```python
from build123d import *

# Parameters (mm, degrees)
EXTRUDE_5_DEPTH = 5.5


with BuildPart() as part:
    # Эскиз1 → Бобышка-Вытянуть5 (new body)
    with BuildSketch(Plane(origin=(0, 0, 0), x_dir=(0, 0, -1), z_dir=(1, 0, 0))):
        Polygon((0.00204272, 35), (0.00204272, 0.000377999), (35.00204272, 0.000377999), (35.00204272, 5.000377999), (70, 5.000377999), (70, 0.000377999), (105.00204272, 0.000377999), (105.00204272, 5.000377999), (140, 5.000377999), (140, 0.000377999), (170, 0.000377999), (170, 35.000377999), (175, 35.000377999), (175, 70), (170, 70), (170, 105.000377999), (175, 105.000377999), (175, 140), (170, 140), (170, 170.000377999), (140.00204272, 170.000377999), (140.00204272, 175.000377999), (139.90204272, 175.000377999), (105, 175.000377999), (105, 170.000377999), (70.00204272, 170.000377999), (70.00204272, 175.000377999), (35, 175.000377999), (35, 170.000377999), (0.00204272, 170.000377999), (0.00204272, 140.000377999), (5.00204272, 140.000377999), (5.00204272, 105), (0.00204272, 105), (0.00204272, 70.000377999), (5.00204272, 70.000377999), (5.00204272, 35), align=None)
        Polygon((71.614687911, 65.697512044), (117.541103017, 19.771096938), (25.688272806, 19.771096938), align=None, mode=Mode.SUBTRACT)
        Polygon((20.031418556, 82.648268821), (48.641577373, 54.038110004), (20.031418556, 25.427951188), align=None, mode=Mode.SUBTRACT)
        Polygon((100.61937762, 42.349676584), (131.978534805, 73.708833769), (155.00204272, 50.685325854), (155.00204272, 19.771096938), (123.197957266, 19.771096938), align=None, mode=Mode.SUBTRACT)
        Polygon((105.802272221, 99.885096353), (129.15010768, 76.537260894), (97.790950495, 45.178103709), (74.443115036, 68.525939168), align=None, mode=Mode.SUBTRACT)
        Polygon((20.031418556, 150.499080414), (82.56698317, 87.963515801), (51.470004498, 56.866537129), (20.031418556, 88.30512307), align=None, mode=Mode.SUBTRACT)
        Polygon((84.688303513, 154.741721101), (117.016745992, 122.413278623), (86.809623857, 92.206156488), (24.274059243, 154.741721101), align=None, mode=Mode.SUBTRACT)
        Polygon((108.630699345, 102.713523478), (155.00204272, 149.084866852), (155.00204272, 56.342180104), align=None, mode=Mode.SUBTRACT)
        Polygon((149.34518847, 154.741721101), (119.845173116, 125.241705748), (90.345157763, 154.741721101), align=None, mode=Mode.SUBTRACT)
    extrude(amount=EXTRUDE_5_DEPTH)


solid = part.part
```
Geometry check sheet. Reference: the model listing, model coordinates, mm. A direction names the side the tool comes from. Coordinates: 2 decimals unless noted, no trailing zeros. Loops run counter-clockwise (first coordinate to the right, second up) from the corner with the lowest first, then second, coordinate; pieces in that order, holes last.
Item 1: Sectioned sample at A-A, the plane z = -62.5. Record the boundary of the cut face in (x, y), then the cut area to 3 significant figures.
Item 2: Sectioned sample at C-C, the plane y = 119.5. Record the boundary of the cut face in (x, z).
Item 3: Release check for a two-part mould opening along Z. For faces 5 (the face through (3, 155, -170)), 6 (the face through (3, 0, -87)), 7 (the face through (2.712, 83.986, -89.903)) record: released by +Z, released by -Z, zero draft, split by the parting line, or undercut.
Item 4: Sectioned sample at B-B, the plane y = 146. Record the boundary of the cut face in (x, z), then the cut area to 3 significant figures.
Item 5: Thickness scan on line 1 (Y direction, x = 5.15, z = -99); line 2 (Y direction, x = 2.9, z = -139); line 3 (Z direction, x = 3.7, y = 150). Record the ranges inside material, lowest first.
Item 6: Sectioned sample at D-D, the plane z = -153. Record the boundary of the cut face in (x, y).
Item 7: Go/stop test with flat-tipped pins: pin 1 Ø1.6 at (x, z) = (2.5, -22) entering from +Y; pin 2 Ø1.6 at (x, y) = (2, 50.5) entering from +Z; pin 3 Ø3 at (y, z) = (103, -108) entering from -X; pin 4 Ø1.5 at (x, y) = (2.5, 172.5) entering from +Z. Record where each tip stops, or that it passes through.
Item 8: Access from +Z, -Z, +X, -X, +Y, -Y to the whole of each face (thin tool, end or side, straight path). Record for faces 1 (the face through (3, 70, -173)), 2 (the face through (3, 5, -52)), 3 (the face through (2.712, 72.633, -67.236)), 4 (the face through (3, 170, -88)).
Check result:
1. outline: (0, 5) - (5.5, 5) - (5.5, 19.77) - (0, 19.77) - close; (0, 56.58) - (5.5, 56.58) - (5.5, 67.9) - (0, 67.9) - close; (0, 108.03) - (5.5, 108.03) - (5.5, 116.52) - (0, 116.52) - close; (0, 154.74) - (5.5, 154.74) - (5.5, 175) - (0, 175) - close
1. area: 302 mm2
2. outline: (0, -175) - (5.5, -175) - (5.5, -155) - (0, -155) - close; (0, -125.42) - (5.5, -125.42) - (5.5, -114.1) - (0, -114.1) - close; (0, -59.52) - (5.5, -59.52) - (5.5, -51.03) - (0, -51.03) - close; (0, -20.03) - (5.5, -20.03) - (5.5, -5) - (0, -5) - close
3. face 5: released by -Z
3. face 6: zero draft
3. face 7: undercut
4. outline: (0, -170) - (5.5, -170) - (5.5, -155) - (0, -155) - close; (0, -151.92) - (5.5, -151.92) - (5.5, -140.6) - (0, -140.6) - close; (0, -99.09) - (5.5, -99.09) - (5.5, -93.43) - (0, -93.43) - close; (0, -33.02) - (5.5, -33.02) - (5.5, -24.53) - (0, -24.53) - close; (0, -20.03) - (5.5, -20.03) - (5.5, 0) - (0, 0) - close
4. area: 333 mm2
5. line 1: y = 0 to 19.77, 38.31 to 46.39, 93.08 to 104.4, 140.43 to 146.09, 154.74 to 170
5. line 2: y = 5 to 19.77, 66.69 to 72.34, 133.08 to 144.4, 154.74 to 175
5. line 3: z = -170 to -144.6, -95.09 to -89.43, -29.02 to -20.53, -20.03 to 0
6. outline: (0, 0) - (5.5, 0) - (5.5, 19.77) - (0, 19.77) - close; (0, 52.69) - (5.5, 52.69) - (5.5, 58.34) - (0, 58.34) - close; (0, 147.08) - (5.5, 147.08) - (5.5, 170) - (0, 170) - close
7. pin 1: stops at y = 170
7. pin 2: stops at z = -5
7. pin 3: stops at x = 0
7. pin 4: stops at z = -35
8. face 1: -Z, +X, -X
8. face 2: +X, -X, -Y
8. face 3: +X, -X
8. face 4: +X, -X, +Y
